```python
from build123d import *

# Parameters (mm, degrees)
SKETCH1_W           = 87.7
SKETCH1_H           = 108
BOSS_EXTRUDE1_DEPTH = 21
SKETCH2_W           = 41.008045073
SKETCH2_H           = 61
CUT_EXTRUDE1_DEPTH  = 11
SKETCH5_W           = 87.7
SKETCH5_H           = 15
CUT_EXTRUDE2_DEPTH  = 16
SKETCH7_W           = 15
SKETCH7_H           = 37
BOSS_EXTRUDE2_DEPTH = 30.9
SKETCH8_W           = 27
SKETCH8_H           = 10.9
CUT_EXTRUDE3_DEPTH  = 30.9


with BuildPart() as part:
    # Sketch1 → Boss-Extrude1 (new body)
    with BuildSketch(Plane(origin=(0, 0, 0), x_dir=(1, 0, 0), z_dir=(0, 1, 0))):
        with Locations((43.85, 54)):
            Rectangle(SKETCH1_W, SKETCH1_H)
    extrude(amount=BOSS_EXTRUDE1_DEPTH)

    # Sketch2 → Cut-Extrude1 (cut)
    with BuildSketch(Plane(origin=(0, 0, 0), x_dir=(-1, 0, 0), z_dir=(0, -1, 0))):
        with Locations((-67.195977464, 30.5)):
            Rectangle(SKETCH2_W, SKETCH2_H)
    extrude(amount=-CUT_EXTRUDE1_DEPTH, mode=Mode.SUBTRACT)

    # Sketch5 → Cut-Extrude2 (cut)
    with BuildSketch(Plane(origin=(0, 21, 0), x_dir=(1, 0, 0), z_dir=(0, 1, 0))):
        with Locations((43.85, 100.5)):
            Rectangle(SKETCH5_W, SKETCH5_H)
    extrude(amount=-CUT_EXTRUDE2_DEPTH, mode=Mode.SUBTRACT)

    # Sketch7 → Boss-Extrude2 (add)
    with BuildSketch(Plane(origin=(0, 21, 0), x_dir=(1, 0, 0), z_dir=(0, 1, 0))):
        with Locations((50.2, 74.5)):
            Rectangle(SKETCH7_W, SKETCH7_H)
    extrude(amount=BOSS_EXTRUDE2_DEPTH)

    # Sketch8 → Cut-Extrude3 (cut)
    with BuildSketch(Plane(origin=(57.7, 0, 0), x_dir=(0, 0, -1), z_dir=(1, 0, 0))):
        with Locations((74.5, 36.45)):
            Rectangle(SKETCH8_W, SKETCH8_H)
    extrude(amount=-CUT_EXTRUDE3_DEPTH, mode=Mode.SUBTRACT)


solid = part.part
```
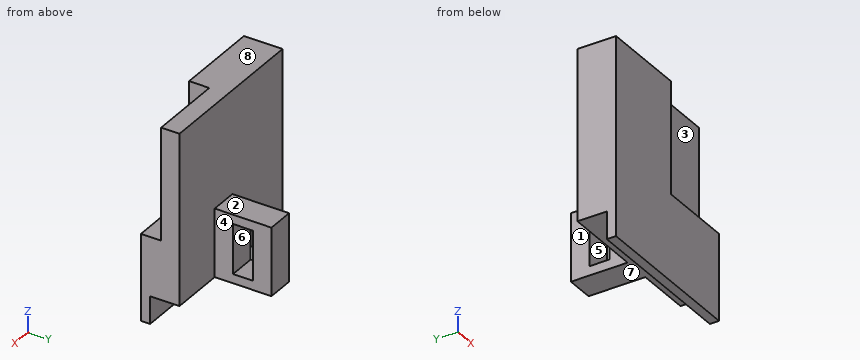
Build history of the part. All positions in model axes, mm. Face numbers are marked on the shaded views. A direction names the side the tool comes from. Round coordinates to 2 decimals unless told otherwise and drop trailing zeros. Order: outer loops, then holes, each group sorted by start corner. A loop starts at its lowest first (then second) coordinate and runs counter-clockwise, first axis right, second up. Notation, with made-up numbers: (62.5, 61.5) - (72.5, 61.5) arc R30 ccw to (72.5, 98.5) - close; hole circle Ø8 at (26.25, 10). An arc over 180 degrees is marked (long way). Use a Markdown table: item, result.
1) Saw through at B-B on x = 52. Write the cut outline in (y, z).
Recorded:
| item | result |
|---|---|
| outline | (0, -108) - (5, -108) - (5, -93) - (51.9, -93) - (51.9, -56) - (21, -56) - (21, 0) - (11, 0) - (11, -61) - (0, -61) - close; hole (31, -88) - (41.9, -88) - (41.9, -61) - (31, -61) - close |
2) Saw through at C-C on x = 9.5. Write the cut outline in (y, z), and give its area (3 significant figures).
Recorded:
| item | result |
|---|---|
| outline | (0, -108) - (5, -108) - (5, -93) - (21, -93) - (21, 0) - (0, 0) - close |
| area | 2,030 mm² |
3) Pull direction Z, two halves, no side cores. Call the marked faces 6, 7 and 8: pulls with the +Z half, pulls with the -Z half, needs draft (parallel to the pull), parting line crosses it, or undercut.
Recorded:
| item | result |
|---|---|
| face 6 | undercut |
| face 7 | pulls with the -Z half |
| face 8 | pulls with the +Z half |
4) Saw through at A-A on z = -69. Write the cut outline in (x, y), and give its area (3 significant figures).
Recorded:
| item | result |
|---|---|
| outline | (0, 0) - (87.7, 0) - (87.7, 21) - (57.7, 21) - (57.7, 31) - (42.7, 31) - (42.7, 21) - (0, 21) - close; (42.7, 41.9) - (57.7, 41.9) - (57.7, 51.9) - (42.7, 51.9) - close |
| area | 2,140 mm² |
5) Wall check: L1, parallel to Y at x = 43.5, z = -80; L2, parallel to Z at x = 44.5, y = 41; L3, parallel to Y at x = 41, z = -4. Give the ranges that are in metal, low to high.
Recorded:
| item | result |
|---|---|
| L1 | y = 0 to 31, 41.9 to 51.9 |
| L2 | z = -93 to -88, -61 to -56 |
| L3 | y = 0 to 21 |
6) Tool access for the marked faces 1, 2, 3, 4 and 5: list every direction of +Z, -Z, +X, -X, +Y, -Y with a clear straight run to the whole face (end or side of a thin tool).
Recorded:
| item | result |
|---|---|
| face 1 | +Z, -Z, -X, +Y |
| face 2 | +Z, +X, -X, +Y |
| face 3 | +Z, +X, -Y |
| face 4 | +Z, -Z, +X, +Y |
| face 5 | +X, -X |
7) Saw through at D-D on y = 7. Write the cut outline in (x, z), and give its area (3 significant figures).
Recorded:
| item | result |
|---|---|
| outline | (0, -93) - (87.7, -93) - (87.7, -61) - (46.69, -61) - (46.69, 0) - (0, 0) - close |
| area | 5,650 mm² |
8) Flat gauge pins, fed straight in: pin 1 Ø5 at (x, y) = (44.5, 17) entering from -Z; pin 2 Ø16.5 at (x, y) = (49, 34.5) entering from +Z; pin 3 Ø1.5 at (x, z) = (75.5, -23.5) entering from -Y. Where does each tip first touch, or does it go through?
Recorded:
| item | result |
|---|---|
| pin 1 | stops at z = -93 |
| pin 2 | stops at z = -56 |
| pin 3 | stops at y = 11 |
